```python
from build123d import *

# Parameters (mm, degrees)
F1_DEPTH      = 2.5
F2_R          = 5
F3_R          = 35
F4_R          = 2
F5_DEPTH      = 2.5
F5_DEPTH_BACK = 2.5


with BuildPart() as f1:
    # F0 (on Front) → F1 (new body, symmetric)
    with BuildSketch(Plane.XZ):
        Polygon((-30, 0), (0, 0), (0, -350.8333333333), (-80, -350.8333333333), (-190, -30), (-190, 0), (-240, 0), (-240, -15), (-220, -15), (-220, -35), (-101.4285714286, -380.8333333333), (30, -380.8333333333), (30, 10), (0, 10), (-30, 5), align=None)
    extrude(amount=F1_DEPTH, both=True)

    # F2
    f2_edges = [f1.edges().sort_by_distance(p)[0] for p in [
        (-240, 0, -15),
        (-220, 0, -15),
        (30, 0, 10),
        (0, 0, 10),
        (0, 0, 0),
        (0, 0, -350.833333),
        (-80, 0, -350.833333),
        (-190, 0, -30),
    ]]
    fillet(f2_edges, radius=F2_R)

    # F3
    f3_edges = [f1.edges().sort_by_distance(p)[0] for p in [
        (-220, 0, -35),
        (-101.428571, 0, -380.833333),
        (30, 0, -380.833333),
    ]]
    fillet(f3_edges, radius=F3_R)

    # F4 (on Front) → F5 (cut, two sides)
    with BuildSketch(Plane.XZ) as f5_sk:
        with Locations((-230, -7.5)):
            Circle(F4_R)
        with Locations((-200, -7.5)):
            Circle(F4_R)
    extrude(amount=F5_DEPTH, mode=Mode.SUBTRACT)
    extrude(f5_sk.sketch, amount=-F5_DEPTH_BACK, mode=Mode.SUBTRACT)


solid = f1.part
```
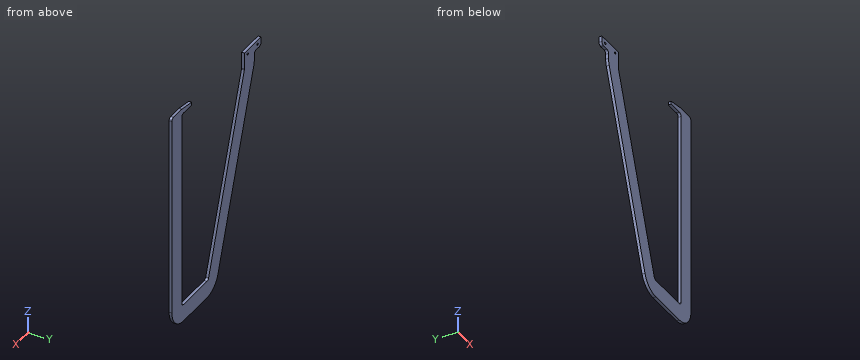
Read the model definition and answer for the solid it produces. Units are mm, in the model's axes. Coordinates: 2 decimals unless noted, no trailing zeros. Loops run counter-clockwise (first coordinate to the right, second up) from the corner with the lowest first, then second, coordinate; pieces in that order, holes last.
(1) The part is cut by section A-A (z = -250). Determine the outline of the cut face in (x, y).
Solution:
outline: (-146.29, -2.5) - (-114.57, -2.5) - (-114.57, 2.5) - (-146.29, 2.5) - close; (0, -2.5) - (30, -2.5) - (30, 2.5) - (0, 2.5) - close
(2) The part is cut by section D-D (x = -132). Determine the outline of the cut face in (y, z).
Solution:
outline: (-2.5, -291.67) - (2.5, -291.67) - (2.5, -199.17) - (-2.5, -199.17) - close
(3) The part is cut by section B-B (y = -0.75). Determine the outline of the cut face in (x, z).
Solution:
outline: (-240, -10) arc R5 ccw to (-235, -15) - (-225, -15) arc R5 cw to (-220, -20) - (-220, -29.17) arc R35 ccw to (-218.11, -40.52) - (-109.54, -357.18) arc R35 ccw to (-76.43, -380.83) - (-5, -380.83) arc R35 ccw to (30, -345.83) - (30, 5) arc R5 ccw to (25, 10) - (0.41, 10) arc R5 ccw to (-0.41, 9.93) - (-30, 5) - (-30, 0) - (-5, 0) arc R5 cw to (0, -5) - (0, -345.83) arc R5 cw to (-5, -350.83) - (-76.43, -350.83) arc R5 cw to (-81.16, -347.45) - (-189.73, -30.79) arc R5 cw to (-190, -29.17) - (-190, 0) - (-240, 0) - close; hole circle Ø4 at (-230, -7.5); hole circle Ø4 at (-200, -7.5)
(4) Flat-ended cylindrical pins translate along their axes: pin 1 Ø2.5 at (x, y) = (-36.5, 1) entering from +Z; pin 2 Ø2.5 at (x, y) = (-202.5, -0.5) entering from +Z. Find the tip coordinate at first contact, or state that the pin passes through.
Solution:
pin 1: stops at z = -350.83
pin 2: stops at z = 0
(5) The part is cut by section C-C (z = -36.5). Determine the outline of the cut face in (x, y), and give its area (3 significant figures).
Solution:
outline: (-219.22, -2.5) - (-187.77, -2.5) - (-187.77, 2.5) - (-219.22, 2.5) - close; (0, -2.5) - (30, -2.5) - (30, 2.5) - (0, 2.5) - close
area: 307 mm2
(6) Consider line 1 along X through (y, z) = (1.7, -58); line 2 along X through (y, z) = (-0.2, -62); line 3 along Z through (x, y) = (-2, -1.4). Determine where each line is inside the solid, lowest interval first.
Solution:
line 1: x = -212.11 to -180.4, 0 to 30
line 2: x = -210.74 to -179.03, 0 to 30
line 3: z = -380.7 to -349.83, -1 to 9.67
